Print and shaded views of the part. All mm, measured from the part's lowest x, y and z. Round coordinates to 2 decimals unless told otherwise and drop trailing zeros. Loops run counter-clockwise (first coordinate to the right, second up) from the corner with the lowest first, then second, coordinate; pieces in that order, holes last. Notation, with made-up numbers: (-18.5, 2) -> (14.5, 2) arc R37 ccw to (14.5, 39) -> close; hole circle Ø5 at (-14, -17). An arc over 180 degrees is marked (long way). Use a Markdown table: item, result.
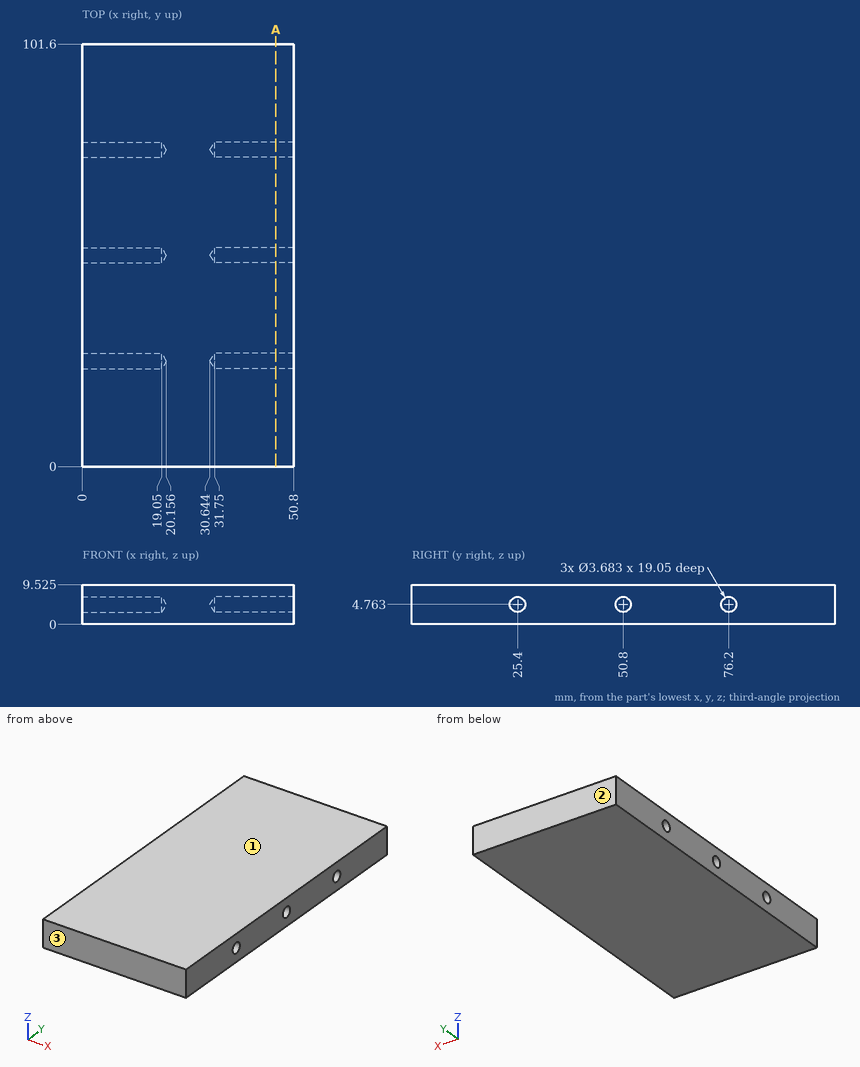
Q1. Pull direction Y, two halves, no side cores. Call the marked faces 1, 2 and 3: released by +Y, released by -Y, zero draft, split by the parting line, or undercut.
Results list:
| item | result |
|---|---|
| face 1 | zero draft |
| face 2 | released by +Y |
| face 3 | released by -Y |
Q2. Flat gauge pin, fed straight in: pin 1 (3 mm diameter, centred on y = 25.4, z = 4.76, fed in from -X) (1 decimal). Where does the tip first touch, or does it go through?
Results list:
| item | result |
|---|---|
| pin 1 | stops at x = 19.3 |
Q3. Band-saw the part on A-A, the plane x = 46.5. Give the cut face in (y, z) (1 decimal).
Results list:
| item | result |
|---|---|
| outline | (0, 0) -> (101.6, 0) -> (101.6, 9.5) -> (0, 9.5) -> close; hole circle Ø3.7 at (25.4, 4.8); hole circle Ø3.7 at (50.8, 4.8); hole circle Ø3.7 at (76.2, 4.8) |
Q4. Drill centre lines: L1, parallel to Z at x = 9.75, y = 25.4 (1 decimal); L2, parallel to Y at x = 18.5, z = 5.5; L3, parallel to Z at x = 36, y = 49.5 (1 decimal). Where is each one in solid material? Low to high. Write a range as from..to.
Results list:
| item | result |
|---|---|
| L1 | z = 0..2.9, 6.6..9.5 |
| L2 | y = 0..23.71, 27.09..49.11, 52.49..74.51, 77.89..101.6 |
| L3 | z = 0..3.5, 6.1..9.5 |
